Geometry check sheet. Reference: the model listing, model coordinates, mm. Round coordinates to 2 decimals unless told otherwise and drop trailing zeros. Loops run counter-clockwise (first coordinate to the right, second up) from the corner with the lowest first, then second, coordinate; pieces in that order, holes last. Notation, with made-up numbers: (-37.75, -5.5) -> (-18.75, -5.5) arc R9 cw to (-18.75, 10.5) -> close; hole circle Ø10 at (55.5, 56.25). An arc over 180 degrees is marked (long way). Use one line per item in the form item = value.
from build123d import *

# Parameters (mm, degrees)
SKETCH1_W           = 105
SKETCH1_H           = 45
BOSS_EXTRUDE1_DEPTH = 3
SKETCH2_R           = 3
SKETCH2_R_2         = 1.5
CUT_EXTRUDE1_DEPTH  = 4
CUT_EXTRUDE2_DEPTH  = 4
FILLET3_R           = 5
SKETCH4_W           = 3
SKETCH4_H           = 5
BOSS_EXTRUDE2_DEPTH = 3
LPATTERN1_COUNT     = 4
LPATTERN1_PITCH     = 30


with BuildPart() as part:
    # Sketch1 → Boss-Extrude1 (new body)
    with BuildSketch(Plane(origin=(0, 0, 0), x_dir=(0, 0, -1), z_dir=(1, 0, 0))):
        with Locations((22.5, 22.5)):
            Rectangle(SKETCH1_W, SKETCH1_H)
    extrude(amount=BOSS_EXTRUDE1_DEPTH)

    # Sketch2 → Cut-Extrude1 (cut, through all)
    with BuildSketch(Plane(origin=(3, 0, 0), x_dir=(0, 0, -1), z_dir=(1, 0, 0))):
        with Locations((6.8, 23.5)):
            Circle(SKETCH2_R)
        with Locations((46.8, 23.5)):
            Circle(SKETCH2_R)
        with Locations((66.8, 38.5)):
            Circle(SKETCH2_R_2)
        with Locations((-13.2, 38.5)):
            Circle(SKETCH2_R_2)
        with BuildLine():
            Line((25.3, 38.5), (25.3, 45))
            Line((25.3, 45), (28.3, 45))
            Line((28.3, 45), (28.3, 38.5))
            ThreePointArc((28.3, 38.5), (26.8, 37), (25.3, 38.5))
        make_face()
    extrude(amount=-CUT_EXTRUDE1_DEPTH, mode=Mode.SUBTRACT)

    # Sketch3 → Cut-Extrude2 (cut, through all)
    with BuildSketch(Plane(origin=(3, 0, 0), x_dir=(0, 0, -1), z_dir=(1, 0, 0))):
        with BuildLine():
            Line((-25, 15), (-30, 15))
            Line((-30, 15), (-30, 18))
            Line((-30, 18), (-25, 18))
            ThreePointArc((-25, 18), (-23.5, 16.5), (-25, 15))
        make_face()
    extrude(amount=-CUT_EXTRUDE2_DEPTH, mode=Mode.SUBTRACT)

    # Fillet3
    fillet3_edges = [part.edges().sort_by_distance(p)[0] for p in [
        (1.5, 45, 30),
        (1.5, 45, -75),
    ]]
    fillet(fillet3_edges, radius=FILLET3_R)

    # Sketch4 → Boss-Extrude2 (add)
    with BuildSketch(Plane(origin=(0, 0, 0), x_dir=(1, 0, 0), z_dir=(0, 1, 0))):
        with Locations((1.5, -22.5)):
            Rectangle(SKETCH4_W, SKETCH4_H)
    boss_extrude2 = extrude(amount=-BOSS_EXTRUDE2_DEPTH)

    # LPattern1: Boss-Extrude2 ×4
    with Locations(*[(0, 0, -i * LPATTERN1_PITCH) for i in range(1, LPATTERN1_COUNT)]):
        add(boss_extrude2)


solid = part.part
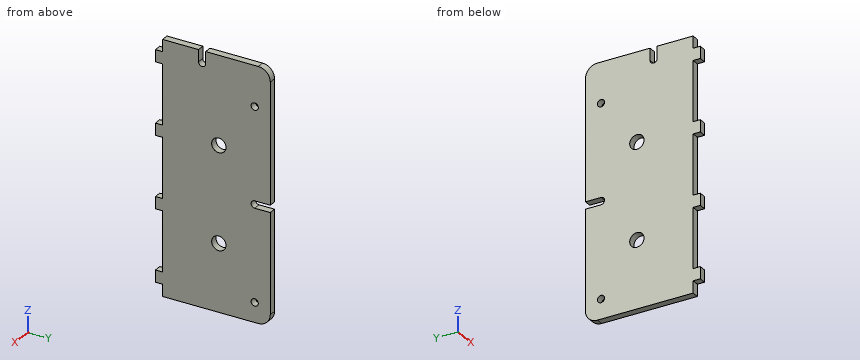
1. Section check A-A (z = -45). Record the boundary of the cut face in (x, y).
Return value:
outline = (0, 0) -> (3, 0) -> (3, 21.1) -> (0, 21.1) -> close; (0, 25.9) -> (3, 25.9) -> (3, 45) -> (0, 45) -> close
2. Section check D-D (z = -26.8). Record the boundary of the cut face in (x, y).
Return value:
outline = (0, 0) -> (3, 0) -> (3, 37) -> (0, 37) -> close
3. Gauge pin test, flat ends, axial feed: pin 1 (0.9 mm diameter, centred on x = 1, y = -1.5, fed in from +Z); pin 2 (0.9 mm diameter, centred on x = 2, y = 41.5, fed in from -Z); pin 3 (0.9 mm diameter, centred on x = 1, z = -71.5, fed in from -Y); pin 4 (5.5 mm diameter, centred on y = 23.5, z = -6.8, fed in from -X). Record the tip position at first contact, or that the pin passes through.
Return value:
pin_1 = 25
pin_2 = -74.89
pin_3 = 0
pin_4 = through
4. Section check B-B (x = 1.2). Count the separate pieces of the cut face and the enclosed holes in it, then the cut area to 3 significant figures.
Return value:
separate_pieces = 1
enclosed_holes = 4
area = 4,660 mm2
5. Section check C-C (z = -6.8). Record the boundary of the cut face in (x, y), then the cut area to 3 significant figures.
Return value:
outline = (0, -3) -> (3, -3) -> (3, 20.5) -> (0, 20.5) -> close; (0, 26.5) -> (3, 26.5) -> (3, 45) -> (0, 45) -> close
area = 126 mm2
6. Material ranges on line 1 along Y through (x, z) = (1.6, -6.8); line 2 along Z through (x, y) = (2.05, 26); line 3 along Z through (x, y) = (2.35, 25), recorded low to high.
Return value:
line_1 = -3 to 20.5, 26.5 to 45
line_2 = -75 to -48.46, -45.14 to -8.46, -5.14 to 30
line_3 = -75 to -49.4, -44.2 to -9.4, -4.2 to 30
